```python
from build123d import *

# Parameters (mm, degrees)
SKETCH_9_R               = 72
SKETCH_9_R_2             = 70
EXTRUDE_9_DEPTH          = 10
SKETCH_9_18_R            = 70
SKETCH_9_18_R_2          = 66
EXTRUDE_10_DEPTH         = 2.5
SKETCH_9_19_R            = 66
EXTRUDE_11_DEPTH         = 10
SHELL_START              = -10
SHELL_2_OUTLINE_R        = 64
SHELL_2_DEPTH            = 8
F_3_0MM_1_REACH          = 163.118
F_3_0MM_1_BORE_R         = 1.5
PATTERN_CIRCULAR_1_COUNT = 4
SKETCH_15_W              = 1
SKETCH_15_H              = 2


# Read off the part's stored shape, not the designer's step: 薄殼2
with BuildPart() as part:
    # 草圖9 → 填料-伸長9 (new body)
    with BuildSketch(Plane(origin=(0, 0, 0), x_dir=(1, 0, 0), z_dir=(0, 1, 0))):
        with Locations(Location((0, 0, 0), (0, 0, 270))):
            Circle(SKETCH_9_R)
        with Locations(Location((0, 0, 0), (0, 0, 270))):
            Circle(SKETCH_9_R_2, mode=Mode.SUBTRACT)
    extrude(amount=-EXTRUDE_9_DEPTH)

    # 草圖9<18> → 填料-伸長10 (add)
    with BuildSketch(Plane(origin=(0, 0, 0), x_dir=(1, 0, 0), z_dir=(0, 1, 0))):
        with Locations(Location((0, 0, 0), (0, 0, 270))):
            Circle(SKETCH_9_18_R)
        with Locations(Location((0, 0, 0), (0, 0, 270))):
            Circle(SKETCH_9_18_R_2, mode=Mode.SUBTRACT)
    extrude(amount=-EXTRUDE_10_DEPTH)

    # 草圖9<19> → 填料-伸長11 (add)
    with BuildSketch(Plane(origin=(0, 0, 0), x_dir=(1, 0, 0), z_dir=(0, 1, 0))):
        with Locations(Location((0, 0, 0), (0, 0, 270))):
            Circle(SKETCH_9_19_R)
    extrude(amount=-EXTRUDE_11_DEPTH)

    # 薄殼2 outline → 薄殼2 (cut)
    with BuildSketch(Plane(origin=(0, 0, 0), x_dir=(1, 0, 0), z_dir=(0, 1, 0)).offset(SHELL_START)):
        Circle(SHELL_2_OUTLINE_R)
    extrude(amount=SHELL_2_DEPTH, mode=Mode.SUBTRACT)

    # Ø3.0mm 定位孔1 bore (on position points) → Ø3.0mm 定位孔1 (cut, up to next)
    with BuildSketch(Plane(origin=(0, -6.25, 72), x_dir=(1, 0, 0), z_dir=(0, 0, 1)), mode=Mode.PRIVATE) as f_3_0mm_1_sk1:
        Circle(F_3_0MM_1_BORE_R)
    f_3_0mm_1_tool1 = extrude(f_3_0mm_1_sk1.sketch, amount=-F_3_0MM_1_REACH, mode=Mode.PRIVATE) & part.part
    f_3_0mm_1 = f_3_0mm_1_tool1.solids().sort_by_distance((0, -6.25, 72))[0]
    add(f_3_0mm_1, mode=Mode.SUBTRACT)

    # 環狀複製排列1: Ø3.0mm 定位孔1 ×4 about axis
    pattern_circular_1_axis = Axis((0, -10, 0), (0, 1, 0))
    for i in range(1, PATTERN_CIRCULAR_1_COUNT):
        add(f_3_0mm_1.rotate(pattern_circular_1_axis, i * 360 / PATTERN_CIRCULAR_1_COUNT), mode=Mode.SUBTRACT)

    # 草圖15 → 除料-旋轉2 (revolve, cut)
    with BuildSketch(Plane(origin=(0, 0, 0), x_dir=(0, 0, -1), z_dir=(1, 0, 0))):
        with Locations((-71.5, -2)):
            Rectangle(SKETCH_15_W, SKETCH_15_H)
    revolve(axis=Axis((0, 0, 0), (0, -1, 0)), mode=Mode.SUBTRACT)


solid = part.part
```
Design review of the part built by this model. Coordinates are the model's own, in mm. A direction names the side the tool comes from. Give positions to 0.01 mm unless a question says otherwise; leave off trailing zeros. Order: outer loops, then holes, each group sorted by start corner. A loop starts at its lowest first (then second) coordinate and runs counter-clockwise, first axis right, second up. Notation, with made-up numbers: (35, 74.5) - (89, 74.5) arc R30 ccw to (89, 100.5) - close; hole circle Ø7 at (-8, 33). An arc over 180 degrees is marked (long way). Use a Markdown table: item, result. Add a question column.
(1) Wall thickness on probe 1 along X at (y, z) = (-4.25, 0); probe 2 along Z at (x, y) = (-1, -6.5); probe 3 along Z at (x, y) = (-47, -8.25): over which ranges is each line inside the solid? List them lowest first. Write a range as [from, to].
(2) Add section A-A on x = 58. Give the boundary of the cut face in (y, z).
(3) Mouldability with a two-part tool opening along X and no side actions: class faces 1 (the face through (48, -1, 53)), 2 (the face through (-1, -2, -1)), 3 (the face through (21.627, -0.493, 68.675)) as +X half, -X half, draft (parallel to the pull), parting line (faces both ways), or undercut.
(4) Machinability: for faces 4 (the face through (48, -3, 53)), 5 (the face through (35, -10, -54)), 6 (the face through (21, -2.5, -63)), which of the approach directions +Z, -Z, +X, -X, +Y, -Y give a long, thin tool a straight path to every point of the face, cutting with its end or side? Answer none if there is none.
(5) Clearance check with flat-ended pins moving along their axes: P1, Ø1, axis at x = 51, z = 30, coming from the -Y side; P2, Ø4, axis at x = -17, y = -4.5, coming from the -Z side; P3, Ø3, axis at y = -3.5, z = 46.5, coming from the -X side (3 decimals). State where each tip first meets the part, or that it passes through.
(6) Add section B-B on z = -29.5. Give the boundary of the cut face in (x, y).
Report:
| question | item | result |
|---|---|---|
| 1 | probe 1 | x = [-72, -70], [-66, -64], [64, 66], [70, 72] |
| 1 | probe 2 | z = [-65.99, -63.99], [63.99, 65.99] |
| 1 | probe 3 | z = [-54.54, -51.87], [-46.34, -43.44], [43.44, 46.34], [51.87, 54.54] |
| 2 | outline | (-10, -42.66) - (-3, -42.66) - (-3, -40.95) - (-1, -40.95) - (-1, -42.66) - (0, -42.66) - (0, 42.66) - (-1, 42.66) - (-1, 40.95) - (-3, 40.95) - (-3, 42.66) - (-10, 42.66) - (-10, 39.19) - (-2.5, 39.19) - (-2.5, 31.5) - (-10, 31.5) - (-10, 27.06) - (-2, 27.06) - (-2, -27.06) - (-10, -27.06) - (-10, -31.5) - (-2.5, -31.5) - (-2.5, -39.19) - (-10, -39.19) - close |
| 3 | face 1 | draft |
| 3 | face 2 | undercut |
| 3 | face 3 | parting line |
| 4 | face 4 | none |
| 4 | face 5 | +Z, -Z, +X, -X, -Y |
| 4 | face 6 | -Y |
| 5 | P1 | stops at y = -2 |
| 5 | P2 | stops at z = -70.42 |
| 5 | P3 | stops at x = -56.205 |
| 6 | outline | (-65.68, -10) - (-63.48, -10) - (-63.48, -2.5) - (-59.04, -2.5) - (-59.04, -10) - (-56.8, -10) - (-56.8, -2) - (56.8, -2) - (56.8, -10) - (59.04, -10) - (59.04, -2.5) - (63.48, -2.5) - (63.48, -10) - (65.68, -10) - (65.68, -3) - (64.58, -3) - (64.58, -1) - (65.68, -1) - (65.68, 0) - (-65.68, 0) - (-65.68, -1) - (-64.58, -1) - (-64.58, -3) - (-65.68, -3) - close |
